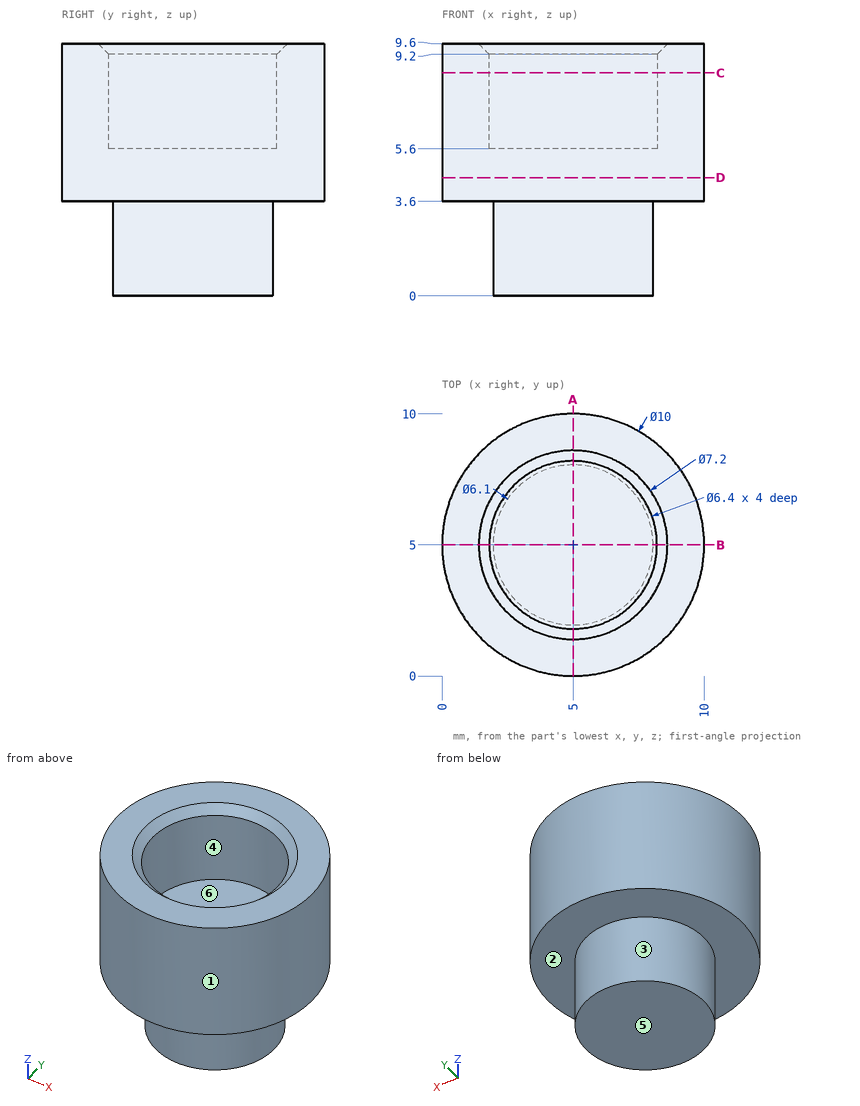
Answer from the drawing. Dimensions are ordinates in mm from the lowest x, y and z of the part. A direction names the side the tool comes from. Coordinates: 2 decimals unless noted, no trailing zeros. Order: outer loops, then holes, each group sorted by start corner. A loop starts at its lowest first (then second) coordinate and runs counter-clockwise, first axis right, second up. Notation, with made-up numbers: (31, 21) - (73, 21) arc R25 ccw to (73, 43) - close; hole circle Ø6 at (70.25, 60.25). An arc over 180 degrees is marked (long way). Answer as a JSON object with one key per item and string values. Group by question number.
Item 1: Section A-A (x = 5) is taken. Give the vertices of the cut face in (y, z).
Item 2: A tool of negligible diameter and unlimited length cuts with its end or side. For the marked faces 1 and 2, from which of +Z, -Z, +X, -X, +Y, -Y can it reach the whole face along a straight path? Write none if from no direction.
Item 3: Section C-C (z = 8.5) is taken. Give the vertices of the cut face in (x, y), plus the area to 3 significant figures.
Item 4: The mould has two halves that part along X. Classify the marked faces 3, 4, 5 and 6: +X half, -X half, draft (parallel to the pull), parting line (faces both ways), or undercut.
Item 5: Flat-ended cylindrical pins translate along their axes: P1, Ø4, axis at x = 5, y = 5, coming from the -Z side; P2, Ø3, axis at x = 3, z = 7.5, coming from the +Y side; P3, Ø1, axis at x = 9, z = 8.5, coming from the -Y side; P4, Ø3, axis at x = 7.5, z = 7.5, coming from the -Y side. Find the tip coordinate at first contact, or state that the pin passes through.
Item 6: Section D-D (z = 4.5) is taken. Give the vertices of the cut face in (x, y), plus the area to 3 significant figures.
Item 7: Consider probe 1 along Y at (x, z) = (5, 8.4); probe 2 along Z at (x, y) = (6.5, 8.75); probe 3 along Z at (x, y) = (4.25, 7). Determine where each line is inside the solid, lowest interval first. Write a range as from..to.
Results are:
{
 "1": {"outline": "(0, 3.6) - (1.95, 3.6) - (1.95, 0) - (8.05, 0) - (8.05, 3.6) - (10, 3.6) - (10, 9.6) - (8.6, 9.6) - (8.2, 9.2) - (8.2, 5.6) - (1.8, 5.6) - (1.8, 9.2) - (1.4, 9.6) - (0, 9.6) - close"},
 "2": {"face 1": "+Z, -Z", "face 2": "-Z"},
 "3": {"outline": "circle Ø10 at (5, 5); hole circle Ø6.4 at (5, 5)", "area": "46.4 mm^2"},
 "4": {"face 3": "parting line", "face 4": "undercut", "face 5": "draft", "face 6": "undercut"},
 "5": {"P1": "stops at z = 0", "P2": "stops at y = 9.97", "P3": "stops at y = 1.43", "P4": "stops at y = 0.1"},
 "6": {"outline": "circle Ø10 at (5, 5)", "area": "78.5 mm^2"},
 "7": {"probe 1": "y = 0..1.8, 8.2..10", "probe 2": "z = 3.6..9.6", "probe 3": "z = 0..5.6"}
}
